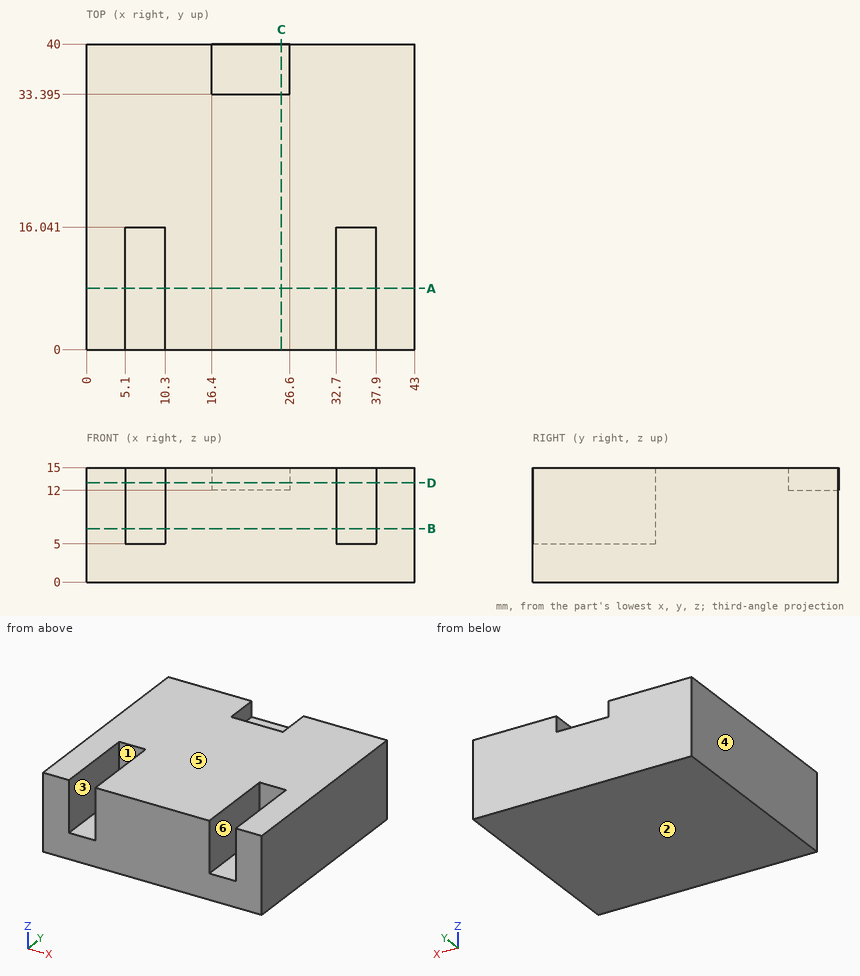
The figure shows three views and two pictorial views of one solid part (mm, origin at its lowest corner). Answer the questions. A direction names the side the tool comes from. Give positions to 0.01 mm unless a question says otherwise; leave off trailing zeros. Write each loop counter-clockwise with the first axis right and the second up, starting at its lowest first coordinate (ties: lowest second). Pieces come first, ordered by that corner, then holes. Notation, with made-up numbers: M 20,-9.5 L 27,-9.5 A11 cw 27,-0.5 Z; hole C 14.5,37 d10. An arc over 180 degrees is marked long. Write each question's results on one line, items separated by ' | '.
Q1. Consider L1, parallel to X at y = 15.5, z = 5.75; L2, parallel to Z at x = 5.5, y = 10; L3, parallel to Y at x = 8, z = 7.5. Determine where each line is inside the solid, lowest interval first. Write a range as from..to.
Output values:
L1: 0..5.1, 10.3..32.7, 37.9..43 | L2: 0..5 | L3: 16.04..40
Q2. A tool of negligible diameter and unlimited length cuts with its end or side. For the marked faces 5 and 6, from which of +Z, -Z, +X, -X, +Y, -Y can it reach the whole face along a straight path? Write none if from no direction.
Output values:
face 5: +Z, +X, -X, +Y, -Y | face 6: +Z, -Y
Q3. Section B-B, the plane z = 7 is taken. Write down the section's boundary in (x, y), then the cut area to 3 significant figures.
Output values:
outline: M 0,0 L 5.1,0 L 5.1,16.04 L 10.3,16.04 L 10.3,0 L 32.7,0 L 32.7,16.04 L 37.9,16.04 L 37.9,0 L 43,0 L 43,40 L 0,40 Z | area: 1,550 mm2
Q4. Section C-C, the plane x = 25.5 is taken. Write down the section's boundary in (y, z) (1 decimal).
Output values:
outline: M 0,0 L 40,0 L 40,12 L 33.4,12 L 33.4,15 L 0,15 Z
Q5. For a pull along X with two mould halves and no side action, classify the marked faces 1, 2, 3 and 4 as released by +X, released by -X, zero draft, split by the parting line, or undercut.
Output values:
face 1: undercut | face 2: zero draft | face 3: undercut | face 4: released by -X
Q6. Section A-A, the plane y = 8 is taken. Write down the section's boundary in (x, z), then the cut area to 3 significant figures.
Output values:
outline: M 0,0 L 43,0 L 43,15 L 37.9,15 L 37.9,5 L 32.7,5 L 32.7,15 L 10.3,15 L 10.3,5 L 5.1,5 L 5.1,15 L 0,15 Z | area: 541 mm2
Q7. Section D-D, the plane z = 13 is taken. Write down the section's boundary in (x, y) (1 decimal), then the cut area to 3 significant figures.
Output values:
outline: M 0,0 L 5.1,0 L 5.1,16 L 10.3,16 L 10.3,0 L 32.7,0 L 32.7,16 L 37.9,16 L 37.9,0 L 43,0 L 43,40 L 26.6,40 L 26.6,33.4 L 16.4,33.4 L 16.4,40 L 0,40 Z | area: 1,490 mm2
Q8. A flat-ended cylindrical pin translates along its axis: P1, Ø2.5, axis at x = 8.5, z = 8.5, coming from the -Y side. Find the tip coordinate at first contact, or state that the pin passes through.
Output values:
P1: y = 16.04
